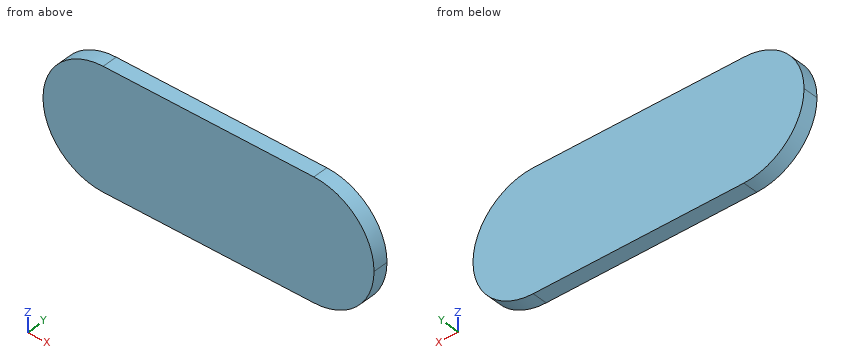
```python
from build123d import *

# Parameters (mm, degrees)
F0_R     = 12.5
F1_DEPTH = 2.5


with BuildPart() as f1:
    # F0 (on Front) → F1 (new body, symmetric)
    with BuildSketch(Plane.XZ):
        with BuildLine():
            ThreePointArc((55, 0), (49.142136, 14.142136), (35, 20))
            Line((35, 20), (-35, 20))
            ThreePointArc((-35, 20), (-49.142136, 14.142136), (-55, 0))
            ThreePointArc((-55, 0), (-49.142136, -14.142136), (-35, -20))
            Line((-35, -20), (35, -20))
            ThreePointArc((35, -20), (49.142136, -14.142136), (55, 0))
        make_face()
        with Locations((35, 0)):
            Circle(F0_R, mode=Mode.SUBTRACT)
        with Locations((35, 0)):
            Circle(F0_R)
    extrude(amount=F1_DEPTH, both=True)


solid = f1.part
```
The model under review builds one solid part; all positions refer to its coordinate system, in mm. Coordinates: 2 decimals unless noted, no trailing zeros. Write each loop counter-clockwise with the first axis right and the second up, starting at its lowest first coordinate (ties: lowest second). Pieces come first, ordered by that corner, then holes. Notation, with made-up numbers: (40.25, -17.75) - (95.25, -17.75) arc R15 cw to (95.25, -13.75) - close; hole circle Ø2 at (-10.75, 67). An arc over 180 degrees is marked (long way). Answer in a Markdown table with one row per item. Add a question column.
Q1. Consider section C-C on x = -38.5. Give the boundary of the cut face in (y, z), then the cut area to 3 significant figures.
Q2. Consider section B-B on z = -11. Give the boundary of the cut face in (x, y), then the cut area to 3 significant figures.
Q3. To check wall thickness, follow line 1 along X through (y, z) = (-0.65, -6.5); line 2 along X through (y, z) = (2, -11); line 3 along Z through (x, y) = (-47, -2.1). State the ranges of each line that lie inside material, in increasing order. Write a range as from..to.
Q4. Clearance check with flat-ended pins moving along their axes: pin 1 (3 mm diameter, centred on y = -1.5, z = 5, fed in from +X); pin 2 (3 mm diameter, centred on y = 0.5, z = 1, fed in from +X); pin 3 (3 mm diameter, centred on y = 1, z = -10, fed in from -X). State where each tip first meets the part, or that it passes through.
Q5. Consider section A-A on y = -0.8. Give the boundary of the cut face in (x, z), then the cut area to 3 significant figures.
Answers below:
| question | item | result |
|---|---|---|
| 1 | outline | (-2.5, -19.69) - (2.5, -19.69) - (2.5, 19.69) - (-2.5, 19.69) - close |
| 1 | area | 197 mm² |
| 2 | outline | (-51.7, -2.5) - (51.7, -2.5) - (51.7, 2.5) - (-51.7, 2.5) - close |
| 2 | area | 517 mm² |
| 3 | line 1 | -53.91..53.91 |
| 3 | line 2 | -51.7..51.7 |
| 3 | line 3 | -16..16 |
| 4 | pin 1 | x = 54.69 |
| 4 | pin 2 | x = 55 |
| 4 | pin 3 | x = -53.1 |
| 5 | outline | (-55, 0) arc R20 ccw to (-35, -20) - (35, -20) arc R20 ccw to (55, 0) arc R20 ccw to (35, 20) - (-35, 20) arc R20 ccw to start |
| 5 | area | 4,060 mm² |
